```python
from build123d import *

# Parameters (mm, degrees)
F1_DEPTH  = 7
F3_DEPTH  = 4.5
F4_R      = 3
F5_R      = 1.49999
F7_D      = 4.4
F10_DEPTH = 3
F11_R     = 2.2
F12_DEPTH = 3
F13_SIZE  = 2.99999


# Not quite as in the source:
# - a fillet or chamfer is up to 0.001 mm smaller than in the source, because OpenCascade refuses the exact size


with BuildPart() as f1:
    # F0 (on Front) → F1 (new body)
    with BuildSketch(Plane.XZ):
        with BuildLine():
            Line((15, -10), (15, 15))
            Line((15, 15), (-15, 15))
            Line((-15, 15), (-15, -10))
            ThreePointArc((-15, -10), (-13.5355339059, -13.5355339059), (-10, -15))
            Line((-10, -15), (10, -15))
            ThreePointArc((10, -15), (13.5355339059, -13.5355339059), (15, -10))
        make_face()
    extrude(amount=F1_DEPTH)

    # F2 (on face) → F3 (join)
    with BuildSketch(Plane.XY.offset(15)):
        with BuildLine():
            Line((-15, 0), (-15, -7))
            Line((-15, -7), (15, -7))
            Line((15, -7), (15, 0))
            Line((15, 0), (15, 15.5))
            ThreePointArc((15, 15.5), (10.6066017178, 26.1066017178), (0, 30.5))
            ThreePointArc((0, 30.5), (-10.6066017178, 26.1066017178), (-15, 15.5))
            Line((-15, 15.5), (-15, 0))
        make_face()
    extrude(amount=-F3_DEPTH)

    # F4
    f4_edges = [f1.edges().sort_by_distance(p)[0] for p in [
        (15, 4.25, 15),
    ]]
    fillet(f4_edges, radius=F4_R)

    # F5 (radius 1.5 in the source; OpenCascade refuses exactly that, so slightly less here)
    f5_edges = [f1.edges().sort_by_distance(p)[0] for p in [
        (15, 7.75, 10.5),
    ]]
    fillet(f5_edges, radius=F5_R)

    # F7 (through all)
    with Locations(Plane.XY.offset(15)):
        with Locations((0, 18)):
            Hole(F7_D / 2)

    # F9 (on offset) → F10 (join)
    with BuildSketch(Plane(origin=(0, 0, -10.5), x_dir=(1, 0, 0), z_dir=(0, 0, -1))):
        with BuildLine():
            Line((12, 0), (-12, 0))
            Line((-12, 0), (-12, -13))
            ThreePointArc((-12, -13), (-8.4852813742, -21.4852813742), (0, -25))
            ThreePointArc((0, -25), (8.4852813742, -21.4852813742), (12, -13))
            Line((12, -13), (12, 0))
        make_face()
    extrude(amount=-F10_DEPTH)

    # F11 (on face) → F12 (cut)
    with BuildSketch(Plane(origin=(0, 0, -10.5), x_dir=(1, 0, 0), z_dir=(0, 0, -1))):
        with Locations((0, -18)):
            Circle(F11_R)
    extrude(amount=-F12_DEPTH, mode=Mode.SUBTRACT)

    # F13 (size 3 in the source; OpenCascade refuses exactly that, so slightly less here)
    f13_edges = [f1.edges().sort_by_distance(p)[0] for p in [
        (-12, 6.5, -7.5),
    ]]
    chamfer(f13_edges, length=F13_SIZE)


solid = f1.part
```
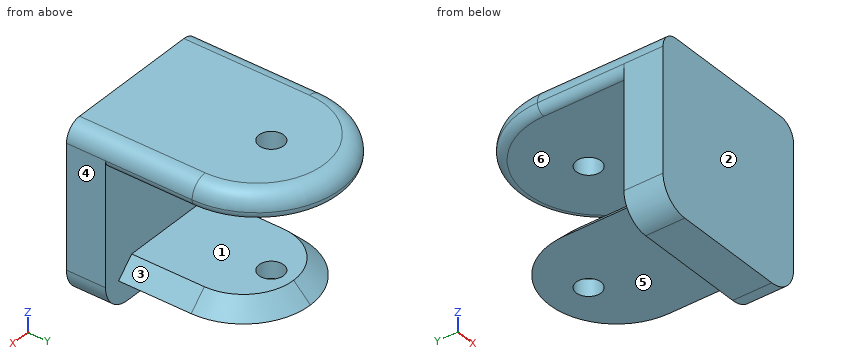
Verification items for the finished model (mm, model axes). Face numbers are marked on the shaded views. A direction names the side the tool comes from. Coordinates: 2 decimals unless noted, no trailing zeros. Loops run counter-clockwise (first coordinate to the right, second up) from the corner with the lowest first, then second, coordinate; pieces in that order, holes last. Notation, with made-up numbers: (-29.5, 80.5) - (-20.5, 80.5) arc R13 ccw to (-20.5, 89.5) - close; hole circle Ø3 at (-8.75, 20.5). An arc over 180 degrees is marked (long way). Put each result on its own line as item: value.
Item 1: Set-up check for the marked faces 1, 2 and 3: record each of +Z, -Z, +X, -X, +Y, -Y from which the full face is reachable in a straight line by a thin tool's end or side.
Conclusion:
face 1: +X, -X, +Y
face 2: +Z, -Z, +X, -X, -Y
face 3: +X, +Y
Item 2: Scan lines: line 1 along Z through (x, y) = (-4, 17.5); line 2 along Y through (x, z) = (-0.25, -6.75); line 3 along Z through (x, y) = (4.75, 22.5). Record each from-to range of solid material in increasing order.
Conclusion:
line 1: z = -10.5 to -7.5, 10.5 to 15
line 2: y = -7 to 0
line 3: z = -10.5 to -9.12, 10.5 to 15
Item 3: Section check B-B (y = 18). Give the number of separate pieces and of enclosed holes in the cut face, then the cut area to 3 significant figures.
Conclusion:
separate pieces: 4
enclosed holes: 0
area: 151 mm2
Item 4: Gauge pin test, flat ends, axial feed: pin 1 Ø1.5 at (x, y) = (-10, 18) entering from -Z; pin 2 Ø6 at (x, z) = (-9.5, -7) entering from +Y; pin 3 Ø8 at (x, z) = (10.5, -1.5) entering from +Y. Record the tip position at first contact, or that the pin passes through.
Conclusion:
pin 1: stops at z = -10.5
pin 2: stops at y = 20.72
pin 3: stops at y = 0
Item 5: Section check A-A (z = 3.5). Enter the section's corners in (x, y).
Conclusion:
outline: (-15, -7) - (15, -7) - (15, 0) - (-15, 0) - close
Item 6: Draft check along Z on the marked faces 4, 5 and 6. Enter one of: pulls with the +Z half, pulls with the -Z half, needs draft (parallel to the pull), parting line crosses it, or undercut.
Conclusion:
face 4: needs draft
face 5: pulls with the -Z half
face 6: undercut
